Part model, mm, in its own coordinate system. Give positions to 0.01 mm unless a question says otherwise; leave off trailing zeros. Order: outer loops, then holes, each group sorted by start corner. A loop starts at its lowest first (then second) coordinate and runs counter-clockwise, first axis right, second up. Notation, with made-up numbers: M 89,54 L 93,54 A6 cw 93,58 Z; hole C 43.25,48 d7. An arc over 180 degrees is marked long. Answer as a JSON object with one key per item and string values.
from build123d import *

# Parameters (mm, degrees)
SKETCH_1_W      = 200
SKETCH_1_H      = 200
SKETCH_1_R      = 3.25
SKETCH_1_R_2    = 1.6
EXTRUDE_1_DEPTH = 3


with BuildPart() as part:
    # 草图1 → 凸台-拉伸1 (new body)
    with BuildSketch(Plane.XY):
        Rectangle(SKETCH_1_W, SKETCH_1_H)
        with Locations((-18.5, 18.5)):
            Circle(SKETCH_1_R, mode=Mode.SUBTRACT)
        with Locations(Location((18.5, 18.5, 0), (0, 0, 180))):
            Circle(SKETCH_1_R, mode=Mode.SUBTRACT)
        with Locations((18.5, -18.5)):
            Circle(SKETCH_1_R, mode=Mode.SUBTRACT)
        with Locations(Location((-18.5, -18.5, 0), (0, 0, 180))):
            Circle(SKETCH_1_R, mode=Mode.SUBTRACT)
        with Locations((97, -50)):
            Circle(SKETCH_1_R_2, mode=Mode.SUBTRACT)
        with Locations(Location((97, 50, 0), (0, 0, 180))):
            Circle(SKETCH_1_R_2, mode=Mode.SUBTRACT)
        with Locations(Location((-97, -50, 0), (0, 0, 180))):
            Circle(SKETCH_1_R_2, mode=Mode.SUBTRACT)
        with Locations((-97, 50)):
            Circle(SKETCH_1_R_2, mode=Mode.SUBTRACT)
        with Locations((-97, 0)):
            Circle(SKETCH_1_R_2, mode=Mode.SUBTRACT)
        with Locations((97, 0)):
            Circle(SKETCH_1_R_2, mode=Mode.SUBTRACT)
    extrude(amount=EXTRUDE_1_DEPTH)


solid = part.part
1. Two-plate mould, pull along Y, no slides. Class faces 1 (the flat face through (-1, 1, 3)), 2 (the cylindrical face through (20.895, 16.303, 1.479)): +Y half, -Y half, draft (parallel to the pull), parting line (faces both ways), or undercut.
Worked answers:
{"face 1": "draft", "face 2": "undercut"}
2. Pin check, flat tip, straight feed: P1, Ø1.9, axis at x = 97, y = 50, coming from the -Z side. Stop position of the tip, or through.
Worked answers:
{"P1": "passes through"}
3. Cut at A-A on x = -18.5. Give the cut face in (y, z), plus the area to 3 significant figures.
Worked answers:
{"outline": "M -100,0 L -21.75,0 L -21.75,3 L -100,3 Z; M -15.25,0 L 15.25,0 L 15.25,3 L -15.25,3 Z; M 21.75,0 L 100,0 L 100,3 L 21.75,3 Z", "area": "561 mm^2"}
4. Probe line 1 along Y through (x, z) = (-18.5, 1.45); line 2 along Y through (x, z) = (-97, 2); line 3 along X through (y, z) = (21, 2.05). List the from-to ranges inside material, lowest first.
Worked answers:
{"line 1": "y = -100 to -21.75, -15.25 to 15.25, 21.75 to 100", "line 2": "y = -100 to -51.6, -48.4 to -1.6, 1.6 to 48.4, 51.6 to 100", "line 3": "x = -100 to -20.58, -16.42 to 16.42, 20.58 to 100"}
